from build123d import *

# Parameters (mm, degrees)
F0_W     = 23.182752
F0_H     = 9.80809
F1_DEPTH = 25.4
F3_DEPTH = 25.4
F4_R     = 6.753053
F5_DEPTH = 25.4


with BuildPart() as f1:
    # F0 (on Front) → F1 (new body)
    with BuildSketch(Plane.XZ):
        with Locations((42.798924, 38.786521)):
            Rectangle(F0_W, F0_H)
    extrude(amount=F1_DEPTH)

    # F2 (on face) → F3 (cut)
    with BuildSketch(Plane.XY.offset(43.690566)):
        with BuildLine():
            ThreePointArc((31.207548, -16.712405), (36.557414, -22.06227), (41.907279, -16.712405))
            ThreePointArc((41.907279, -16.712405), (36.557414, -11.36254), (31.207548, -16.712405))
        make_face()
    extrude(amount=F3_DEPTH, mode=Mode.SUBTRACT)

    # F4 (on face) → F5 (cut)
    with BuildSketch(Plane.XY.offset(43.690566)):
        with Locations((47.316056, -8.88319)):
            Circle(F4_R)
    extrude(amount=-F5_DEPTH, mode=Mode.SUBTRACT)


solid = f1.part
The listing builds one solid part. Answer for the finished solid, in the listing's coordinates (mm). Give positions to 0.01 mm unless a question says otherwise; leave off trailing zeros. Order: outer loops, then holes, each group sorted by start corner. A loop starts at its lowest first (then second) coordinate and runs counter-clockwise, first axis right, second up. Notation, with made-up numbers: (76.25, 77.5) - (88.25, 77.5) arc R13 cw to (88.25, 85.5) - close; hole circle Ø9 at (35.25, -20). An arc over 180 degrees is marked (long way). Answer as CSV lines item,"result".
Q1. Straight lines are drawn through the part: L1, parallel to X at y = -8.75, z = 39.75; L2, parallel to Y at x = 47.25, z = 42; L3, parallel to Y at x = 45.25, z = 40. For each, find the intervals that lie inside material, in ascending order.
Answer key:
L1,"x = 31.21 to 40.56, 54.07 to 54.39"
L2,"y = -25.4 to -15.64, -2.13 to 0"
L3,"y = -25.4 to -15.31, -2.45 to 0"
Q2. Each of these flat-tipped pins is pushed along its axis until it touches: pin 1 Ø11 at (x, y) = (47.32, -8.88) entering from -Z; pin 2 Ø2 at (x, z) = (40, 35) entering from +Y. Where does it stop, or does it pass through?
Answer key:
pin 1,"passes through"
pin 2,"stops at y = 0"
Q3. A cutting plane is placed at C-C, the plane z = 37.25. Determine the outline of the cut face in (x, y).
Answer key:
outline,"(31.21, -25.4) - (54.39, -25.4) - (54.39, 0) - (31.21, 0) - close; hole circle Ø13.51 at (47.32, -8.88)"
Q4. A cutting plane is placed at B-B, the plane x = 47.75. Determine the outline of the cut face in (y, z), and give its area (3 significant figures).
Answer key:
outline,"(-25.4, 33.88) - (-15.62, 33.88) - (-15.62, 43.69) - (-25.4, 43.69) - close; (-2.14, 33.88) - (0, 33.88) - (0, 43.69) - (-2.14, 43.69) - close"
area,"117 mm^2"
Q5. A cutting plane is placed at A-A, the plane y = -14.75. Determine the outline of the cut face in (x, z), and give its area (3 significant figures).
Answer key:
outline,"(31.21, 33.88) - (43.97, 33.88) - (43.97, 43.69) - (31.21, 43.69) - close; (50.66, 33.88) - (54.39, 33.88) - (54.39, 43.69) - (50.66, 43.69) - close"
area,"162 mm^2"
Q6. Determine the mould class of faces 1 (the face through (40.57, -8.59, 38.86)), 2 (the face through (31.208, -13, 39)), 3 (the face through (40, -13, 33.882)) for opening direction X: pulls with the +X half, pulls with the -X half, needs draft (parallel to the pull), parting line crosses it, or undercut.
Answer key:
face 1,"undercut"
face 2,"pulls with the -X half"
face 3,"needs draft"
